For this review, take the finished solid that the model builds, in its own axes (mm). A direction names the side the tool comes from. Coordinates: 2 decimals unless noted, no trailing zeros. Order: outer loops, then holes, each group sorted by start corner. A loop starts at its lowest first (then second) coordinate and runs counter-clockwise, first axis right, second up. Notation, with made-up numbers: (77, 56) -> (136, 56) arc R18 cw to (136, 81) -> close; hole circle Ø9 at (34.5, -38). An arc over 180 degrees is marked (long way). Return JSON: item names as keys, results as strings. Group by question number.
Item 1: Draft analysis for pull direction X (two halves, no side actions). For faces 1 (the flat face through (-137.03, -141.5, 128.43)), 2 (the flat face through (-129.81, -154.01, 128.43)), 3 (the flat face through (-135.21, -156.35, 128.43)), state which applies: +X half, -X half, draft (parallel to the pull), parting line (faces both ways), or undercut.
Item 2: Insertion check: pin 1 (4.5 mm diameter, centred on x = -134.52, y = -148.39, fed in from -Z); pin 2 (1 mm diameter, centred on x = -133, z = 128, fed in from -Y). Each pin has a flat end and moves straight along its axis. Give the tip position at first contact, or say it passes through.
Item 3: Take a section at C-C (y = -142.5). Write out the cut boundary in (x, z).
Item 4: Take a section at A-A (x = -139.25). Write out the cut boundary in (y, z), then the cut area to 3 significant figures.
Item 5: Take a section at D-D (y = -154). Write out the cut boundary in (x, z).
Item 6: Take a section at B-B (y = -147.5). Write out the cut boundary in (x, z).
Item 7: Machinability: for faces 4 (the flat face through (-140.145, -143.674, 128.429)), 5 (the flat face through (-135.8, -141.16, 128.43)), 6 (the flat face through (-130, -143, 128)), which of the approach directions +Z, -Z, +X, -X, +Y, -Y give a long, thin tool a straight path to every point of the face, cutting with its end or side? Answer none if there is none.
Item 8: For line 1 along Y through (x, z) = (-139, 128.1); line 2 along Y through (x, z) = (-139.25, 127.75); line 3 along X through (y, z) = (-143.75, 129.2), list the stretches that pass through material, from the lowest coordinate up.
Autodesk Inventor part; units mm, degrees
ref_plane "YZ Plane" through (0, 0, 0) normal (1, 0, 0) x (0, 1, 0)
ref_plane "XZ Plane" through (0, 0, 0) normal (0, 1, 0) x (-1, 0, 0)
ref_plane "XY Plane" through (0, 0, 0) normal (0, 0, 1) x (1, 0, 0)
ref_plane "Work Plane1" through (-89.269, -103.4593, 127.4153) normal (0, 0, 1) x (0, -1, 0)
sketch "Sketch1" plane through (-89.269, -103.4593, 127.4153) normal (0, 0, 1) x (0, -1, 0)
  circle A0 centre (44.9313, -45.255) radius 1.4 construction
  circle A1 centre (44.9313, -45.255) radius 1.7
  circle A2 centre (44.9313, -45.255) radius 6.7
  point P0 (-103.4593, 89.269)
  dimension "d0" = 0.3
  dimension "d1" = 5
extrude "Extrusion1" add sketch "Sketch1" along normal blind 2
sketch "Sketch2" plane through (-134.524, -148.3906, 129.4153) normal (0, 0, 1) x (1, 0, 0)
  circle A0 centre (0, 0) radius 1.7
  circle A1 centre (0, 0) radius 6.7
  line L0 (-6.7, 0) -> (-8.0802, 0)
  line L1 (-8.0802, 0) -> (-7.8365, -1.3818)
  line L2 (-7.8365, -1.3818) -> (-6.5982, -1.1634)
  circle A2 centre (0, 0) radius 6.7
  line L3 (0, 0) -> (-6.5982, -1.1634)
  line L4 (0, 0) -> (-6.7, 0)
  line L5 (0, 0) -> (6.7, 0) construction
  line L6 (-8.0802, 0) -> (-7.8365, 1.3818)
  line L7 (-7.8365, 1.3818) -> (-6.5982, 1.1634)
  arc A3 (-6.5982, 1.1634) -> (-6.5982, -1.1634) centre (0, 0) ccw
  point P0 (134.524, 148.3906)
  dimension "d4" = 180
  dimension "d7" = 10
extrude "Extrusion2" add sketch "Sketch2" against normal up to surface (2 mm away) contours L0 L6 L7 A1 | A1 L2 L1 L0
pattern_circular "Circular Pattern1" count 12 over 360 about axis through (-134.524, -148.3906, 127.4153) along (0, 0, 1) of "Extrusion2"
sketch "Sketch3" plane through (-89.269, -103.4593, 129.4153) normal (0, 0, 1) x (1, 0, 0)
  circle A0 centre (-45.255, -44.9313) radius 2.45
  line L0 (-42.7892, -48.1333) -> (-46.7952, -48.6677)
  line L1 (-46.7952, -48.6677) -> (-49.261, -45.4657)
  line L2 (-49.261, -45.4657) -> (-47.7208, -41.7292)
  line L3 (-47.7208, -41.7292) -> (-43.7148, -41.1948)
  line L4 (-43.7148, -41.1948) -> (-41.249, -44.3969)
  line L5 (-41.249, -44.3969) -> (-42.7892, -48.1333)
  point P0 (89.269, 103.4593)
  dimension "d11" = 7
extrude "Extrusion3" cut sketch "Sketch3" against normal blind 1.5 contours A0 | L0 L1 L2 L3 L4 L5
properties part number "cellSTORM_screw_ring_adjuster"
Findings below:
{
 "1": {"face 1": "undercut", "face 2": "+X half", "face 3": "-X half"},
 "2": {"pin 1": "stops at z = 127.42", "pin 2": "stops at y = -156.29"},
 "3": {"outline": "(-139.47, 127.42) -> (-129.58, 127.42) -> (-129.58, 129.42) -> (-139.47, 129.42) -> close"},
 "4": {"outline": "(-154.81, 127.42) -> (-154.02, 127.42) -> (-154.02, 129.42) -> (-154.81, 129.42) -> close; (-153.14, 127.42) -> (-143.64, 127.42) -> (-143.64, 129.42) -> (-153.14, 129.42) -> close; (-142.76, 127.42) -> (-141.97, 127.42) -> (-141.97, 129.42) -> (-142.76, 129.42) -> close", "area": "22.2 mm2"},
 "5": {"outline": "(-139.23, 127.42) -> (-129.82, 127.42) -> (-129.82, 129.42) -> (-139.23, 129.42) -> close"},
 "6": {"outline": "(-142.45, 127.42) -> (-135.97, 127.42) -> (-135.97, 127.92) -> (-137.94, 127.92) -> (-137.94, 129.42) -> (-142.45, 129.42) -> close; (-133.08, 127.42) -> (-126.6, 127.42) -> (-126.6, 129.42) -> (-130.79, 129.42) -> (-130.79, 127.92) -> (-133.08, 127.92) -> close"},
 "7": {"face 4": "+Z, -Z, +Y", "face 5": "+Z, -Z", "face 6": "+Z, -Z, +X"},
 "8": {"line 1": "y = -155.02 to -153.72, -153.38 to -143.41, -143.06 to -141.76", "line 2": "y = -154.81 to -154.02, -153.14 to -143.64, -142.76 to -141.97", "line 3": "x = -141.02 to -140.05, -139.36 to -129.69, -128.99 to -128.03"}
}
